from build123d import *

# Parameters (mm, degrees)
SKETCH_1_W      = 238.4
SKETCH_1_H      = 88
EXTRUDE_1_DEPTH = 5.8
SKETCH_2_W      = 5.8
SKETCH_2_H      = 30
SKETCH_2_W_2    = 47.2
SKETCH_2_H_2    = 5.8
EXTRUDE_2_DEPTH = 5.8


with BuildPart() as part:
    # Эскиз1 → Бобышка-Вытянуть1 (new body)
    with BuildSketch(Plane.XY):
        with Locations((119.2, 44)):
            Rectangle(SKETCH_1_W, SKETCH_1_H)
    extrude(amount=EXTRUDE_1_DEPTH)

    # Эскиз2 → Бобышка-Вытянуть2 (add)
    with BuildSketch(Plane.XY.offset(5.8)):
        with Locations((-2.9, 44)):
            Rectangle(SKETCH_2_W, SKETCH_2_H)
        with Locations((241.3, 44)):
            Rectangle(SKETCH_2_W, SKETCH_2_H)
        with Locations((71.6, 90.9)):
            Rectangle(SKETCH_2_W_2, SKETCH_2_H_2)
        with Locations((166.8, 90.9)):
            Rectangle(SKETCH_2_W_2, SKETCH_2_H_2)
        with Locations((71.6, -2.9)):
            Rectangle(SKETCH_2_W_2, SKETCH_2_H_2)
        with Locations((166.8, -2.9)):
            Rectangle(SKETCH_2_W_2, SKETCH_2_H_2)
    extrude(amount=-EXTRUDE_2_DEPTH)


solid = part.part
Work out the finished part from the listing and answer in its coordinate system (mm). A direction names the side the tool comes from. Round coordinates to 2 decimals unless told otherwise and drop trailing zeros. Write each loop counter-clockwise with the first axis right and the second up, starting at its lowest first coordinate (ties: lowest second). Pieces come first, ordered by that corner, then holes.
1) Straight lines are drawn through the part: line 1 (X direction, y = 89, z = 4.4); line 2 (X direction, y = 74, z = 1.45); line 3 (Y direction, x = 135.5, z = 4.1). For each, find the intervals that lie inside material, in ascending order.
2) A cutting plane is placed at A-A (z = 1.15). Give the vertices of the cut face in (x, y), plus the area to 3 significant figures.
3) The mould has two halves that part along X. Classify faces 6 (the flat face through (241, 59, 3)), 7 (the flat face through (119, 88, 3)), 8 (the flat face through (48, 91, 3)), 9 (the flat face through (238.4, 14, 3)): pulls with the +X half, pulls with the -X half, needs draft (parallel to the pull), parting line crosses it, or undercut.
4) Given pin 1 Ø1.7 at (y, z) = (72.5, 3) entering from -X; pin 2 Ø1 at (x, z) = (107.5, 2.5) entering from +Y; pin 3 Ø1.7 at (y, z) = (-2, 3.5) entering from +X, each flat-ended and moving along its own axis, determine where each tip first touches the part or whether it passes through.
5) A cutting plane is placed at C-C (x = 45.5). Give the vertices of the cut face in (y, z), plus the area to 3 significant figures.
6) A cutting plane is placed at B-B (y = 23). Give the vertices of the cut face in (x, z).
7) A tool of negligible diameter and unlimited length cuts with its end or side. For faces 1 (the flat face through (190.4, -3, 3)), 2 (the flat face through (214, 88, 3)), 3 (the flat face through (-3, 59, 3)), 4 (the flat face through (-3, 29, 3)), 5 (the flat face through (143.2, 91, 3)), from which of +Z, -Z, +X, -X, +Y, -Y can it reach the whole face along a straight path? Write none if from no direction.
Completed:
1. line 1: x = 48 to 95.2, 143.2 to 190.4
1. line 2: x = 0 to 238.4
1. line 3: y = 0 to 88
2. outline: (-5.8, 29) - (0, 29) - (0, 0) - (48, 0) - (48, -5.8) - (95.2, -5.8) - (95.2, 0) - (143.2, 0) - (143.2, -5.8) - (190.4, -5.8) - (190.4, 0) - (238.4, 0) - (238.4, 29) - (244.2, 29) - (244.2, 59) - (238.4, 59) - (238.4, 88) - (190.4, 88) - (190.4, 93.8) - (143.2, 93.8) - (143.2, 88) - (95.2, 88) - (95.2, 93.8) - (48, 93.8) - (48, 88) - (0, 88) - (0, 59) - (-5.8, 59) - close
2. area: 22,400 mm2
3. face 6: needs draft
3. face 7: undercut
3. face 8: pulls with the -X half
3. face 9: pulls with the +X half
4. pin 1: stops at x = 0
4. pin 2: stops at y = 88
4. pin 3: stops at x = 190.4
5. outline: (0, 0) - (88, 0) - (88, 5.8) - (0, 5.8) - close
5. area: 510 mm2
6. outline: (0, 0) - (238.4, 0) - (238.4, 5.8) - (0, 5.8) - close
7. face 1: +Z, -Z, +X, -Y
7. face 2: +Z, -Z, +X, +Y
7. face 3: +Z, -Z, -X, +Y
7. face 4: +Z, -Z, -X, -Y
7. face 5: +Z, -Z, +Y
